Build history of the part. All positions in model axes, mm. A direction names the side the tool comes from. Give positions to 0.01 mm unless a question says otherwise; leave off trailing zeros. Write each loop counter-clockwise with the first axis right and the second up, starting at its lowest first coordinate (ties: lowest second). Pieces come first, ordered by that corner, then holes. Notation, with made-up numbers: M -30,47.5 L -22,47.5 A13 ccw -22,60.5 Z; hole C 74.5,25.5 d9. An arc over 180 degrees is marked long. Return JSON: item names as keys, results as strings. Group by question number.
Q1. Band-saw the part on A-A, the plane y = 3.5. Give the cut face in (x, z), then the cut area to 3 significant figures.
Q2. Wall check: probe 1 along Z at (x, y) = (131.5, 2.5); probe 2 along X at (y, z) = (3.9, -270); probe 3 along Z at (x, y) = (-220, 6.5). Give the ranges that are in metal, low to high.
Q3. Pull direction X, two halves, no side cores. Call faces 1 (the flat face through (248.625, 8.244, 263.403)), 2 (the flat face through (-4, 0, -9)), 3 (the flat face through (-27.626, 4.93, -275.21)): +X half, -X half, draft (parallel to the pull), parting line (faces both ways), or undercut.
Q4. Band-saw the part on D-D, the plane x = 224. Give the cut face in (y, z).
Q5. Band-saw the part on C-C, the plane x = 98.5. Give the cut face in (y, z).
Q6. Band-saw the part on B-B, the plane z = -270. Give the cut face in (x, y).
Q7. Tool access for faces 4 (the flat face through (227.916, 4.93, 269.86)), 5 (the flat face through (244.229, 8.292, 267.486)), 6 (the cylindrical face through (250.615, 2.712, 269.951)): list every direction of +Z, -Z, +X, -X, +Y, -Y with a clear straight run to the whole face (end or side of a thin tool).
Q8. Flat gauge pins, fed straight in: pin 1 Ø7.5 at (x, z) = (246.39, 265.34) entering from -Y; pin 2 Ø1 at (x, y) = (29.5, 8.5) entering from -Z; pin 3 Ø10 at (x, z) = (2.5, -271.5) entering from -Y; pin 4 Ø5 at (x, y) = (195, 4) entering from -Z. Where does each tip first touch, or does it go through?
from build123d import *

# Parameters (mm, degrees)
BOSS_EXTRUDE1_DEPTH  = 10
CUT_EXTRUDE1_DEPTH   = 20
FILLET1_R            = 3
FILLET1_OF_MIRROR1_R = 3
CUT_EXTRUDE2_DEPTH   = 20
FILLET2_R            = 3
SKETCH7_R            = 6.25
CUT_EXTRUDE3_DEPTH   = 5.5


with BuildPart() as part:
    # Sketch1 → Boss-Extrude1 (new body)
    with BuildSketch(Plane(origin=(0, 0, 0), x_dir=(1, 0, 0), z_dir=(0, 1, 0))):
        Polygon((-260, -260), (-260, -280), (-240, -280), (-216.164928148, -260), (216.164928148, -260), (240, -280), (260, -280), (260, -260), (260, 260), (45.752607778, 260), (10, 290), (-10, 290), (-45.752607778, 260), (-260, 260), align=None)
    extrude(amount=BOSS_EXTRUDE1_DEPTH)

    # Sketch5 → Cut-Extrude1 (cut)
    with BuildSketch(Plane(origin=(-253.195489006, 0, 272.672065084), x_dir=(0, -1, 0), z_dir=(0.6804510993672804, 0, -0.7327934916262968))):
        Polygon((-10, 6), (-10, -6), (-6.535898385, 0), align=None)
    cut_extrude1 = extrude(amount=CUT_EXTRUDE1_DEPTH, mode=Mode.SUBTRACT)

    # Fillet1
    fillet1_edges = [part.edges().sort_by_distance(p)[0] for p in [
        (-241.784847494, 8.267949192, 255.974841953),
        (-237.388086544, 8.267949192, 260.057548549),
        (-250.997108531, 8.267949192, 274.713418382),
        (-255.393869481, 8.267949192, 270.630711786),
    ]]
    fillet(fillet1_edges, radius=FILLET1_R - 0.0001)  # a hair under: the kernel refuses the full size

    # Mirror1: Cut-Extrude1 across plane
    add(cut_extrude1.mirror(Plane(origin=(0, 0, 0), x_dir=(0, 0, 1), z_dir=(1, 0, 0))), mode=Mode.SUBTRACT)

    # Fillet1 of Mirror1
    fillet1_of_mirror1_edges = [part.edges().sort_by_distance(p)[0] for p in [
        (241.784847494, 8.267949192, 255.974841953),
        (237.388086544, 8.267949192, 260.057548549),
        (250.997108531, 8.267949192, 274.713418382),
        (255.393869481, 8.267949192, 270.630711786),
    ]]
    fillet(fillet1_of_mirror1_edges, radius=FILLET1_OF_MIRROR1_R - 0.0001)  # a hair under: the kernel refuses the full size

    # Sketch6 → Cut-Extrude2 (cut)
    with BuildSketch(Plane(origin=(0, 0, -280), x_dir=(-1, 0, 0), z_dir=(0, 0, -1))):
        Polygon((-6, 10), (6, 10), (0, 6.535898385), align=None)
    extrude(amount=-CUT_EXTRUDE2_DEPTH, mode=Mode.SUBTRACT)

    # Fillet2
    fillet2_edges = [part.edges().sort_by_distance(p)[0] for p in [
        (3, 8.267949192, -260),
        (-3, 8.267949192, -260),
        (3, 8.267949192, -280),
        (-3, 8.267949192, -280),
    ]]
    fillet(fillet2_edges, radius=FILLET2_R - 0.0001)  # a hair under: the kernel refuses the full size

    # Sketch7 → Cut-Extrude3 (cut)
    with BuildSketch(Plane.XZ):
        with Locations(Location((-246.390978013, 265.344130167, 0), (0, 0, 270))):
            Circle(SKETCH7_R)
        with Locations(Location((246.390978013, 265.344130167, 0), (0, 0, 270))):
            Circle(SKETCH7_R)
        with Locations(Location((0, -270, 0), (0, 0, 270))):
            Circle(SKETCH7_R)
    extrude(amount=-CUT_EXTRUDE3_DEPTH, mode=Mode.SUBTRACT)


solid = part.part
From the geometry:
{
 "1": {"outline": "M -260,-260 L -45.75,-260 L -10,-290 L 10,-290 L 45.75,-260 L 260,-260 L 260,280 L 240,280 L 216.16,260 L -216.16,260 L -240,280 L -260,280 Z; hole C -246.39,265.34 d12.5; hole C 0,-270 d12.5; hole C 246.39,265.34 d12.5", "area": "273,000 mm^2"},
 "2": {"probe 1": "z = -260 to 260", "probe 2": "x = -33.84 to -6.25, 6.25 to 33.84", "probe 3": "z = -260 to 263.22"},
 "3": {"face 1": "undercut", "face 2": "draft", "face 3": "-X half"},
 "4": {"outline": "M 0,-260 L 10,-260 L 10,266.57 L 0,266.57 Z"},
 "5": {"outline": "M 0,-260 L 10,-260 L 10,260 L 0,260 Z"},
 "6": {"outline": "M -33.84,0 L -6.25,0 L -6.25,5.5 L 6.25,5.5 L 6.25,0 L 33.84,0 L 33.84,10 L 6,10 L 0,6.54 L -6,10 L -33.84,10 Z"},
 "7": {"face 4": "+Z, +Y, -Y", "face 5": "+Y", "face 6": "-Y"},
 "8": {"pin 1": "stops at y = 5.5", "pin 2": "stops at z = -274.06", "pin 3": "stops at y = 0", "pin 4": "stops at z = -260"}
}
